Input: part model. Units: mm. Frame: model coordinates. Face numbers are marked on the shaded views. A direction names the side the tool comes from. Give positions to 0.01 mm unless a question says otherwise; leave off trailing zeros. Loops run counter-clockwise (first coordinate to the right, second up) from the corner with the lowest first, then second, coordinate; pieces in that order, holes last. Notation, with made-up numbers: (76, 9.25) - (113, 9.25) arc R26 ccw to (113, 31.25) - close; hole circle Ø5 at (40.25, 46.5). An arc over 180 degrees is marked (long way). Answer as a JSON object with one key per item and string values. Group by question number.
(1) Material intervals for L1, parallel to X at y = 26, z = 15.5; L2, parallel to X at y = 38, z = 19.5; L3, parallel to X at y = 38.2, z = 19.5, sorted ascending.
(2) Section query A-A (x = -10). Return loops of the section in (y, z), plus the area to 3 significant figures.
(3) Mould query, pull axis X, two halves, no side actions, for the marked faces 3, 4 and 5. Classes: +X half, -X half, draft (parallel to the pull), parting line (faces both ways), or undercut.
(4) Section query D-D (x = 10). Return loops of the section in (y, z).
(5) Access query for the marked faces 1 and 2. Directions: +Z, -Z, +X, -X, +Y, -Y. A direction counts if a zero-diameter tool reaches every point of the face in a straight line with its end or side. Return the directions, or none.
(6) Pin query (flat end, axial travel): P1, Ø2, axis at x = 12, z = 26.5, coming from the +Y side; P2, Ø0.8, axis at y = -4, z = 13.5, coming from the +X side; P3, Ø1.1, axis at x = 8, z = 13.5, coming from the -Y side; P4, Ø0.6, axis at x = 11.5, z = 27, coming from the -Y side. Return the tip coordinate at first contact, or that it passes through.
(7) Section query C-C (z = 19.5). Return loops of the section in (x, y), plus the area to 3 significant figures.
(8) Section query B-B (y = -18.5). Return loops of the section in (x, z), plus the area to 3 significant figures.
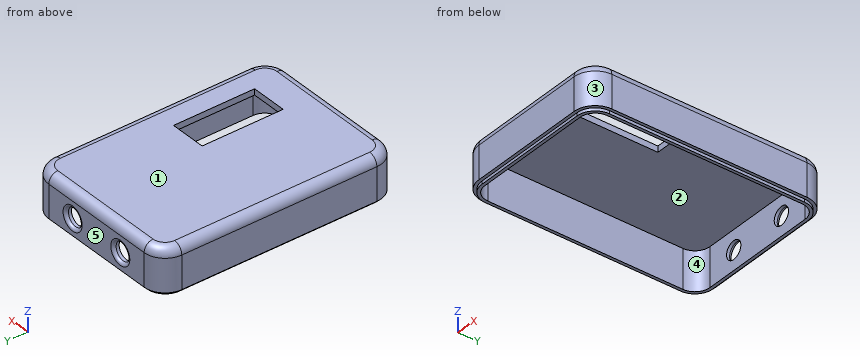
```python
from build123d import *

# Parameters (mm, degrees)
PAD002_DEPTH            = 2
PAD003_DEPTH            = 12
FILLET001_R             = 3
SKETCH006_R             = 3
POCKET002_DEPTH         = 5
PAD004_DEPTH            = 1
FILLET003_R             = 1
SKETCH018_W             = 12
SKETCH018_H             = 27
POCKET004_DEPTH         = 5
BODY001_PLACEMENT_ANGLE = 180


with BuildPart() as part:
    # Sketch003 → Pad002 (new body)
    with BuildSketch(Plane.XY):
        with BuildLine():
            Line((-27, 32.5), (-27, -32.5))
            ThreePointArc((-27, -32.5), (-24.949747, -37.449747), (-20, -39.5))
            Line((-20, -39.5), (20, -39.5))
            ThreePointArc((20, -39.5), (24.949747, -37.449747), (27, -32.5))
            Line((27, -32.5), (27, 32.5))
            ThreePointArc((27, 32.5), (24.949747, 37.449747), (20, 39.5))
            Line((20, 39.5), (-20, 39.5))
            ThreePointArc((-20, 39.5), (-24.949747, 37.449747), (-27, 32.5))
        make_face()
    extrude(amount=PAD002_DEPTH)

    # Sketch004 (on Face10 of Pad002) → Pad003 (join)
    with BuildSketch(Plane.XY.offset(2)):
        with BuildLine():
            Line((-27, 32.5), (-27, -32.5))
            ThreePointArc((-27, -32.5), (-24.949747, -37.449747), (-20, -39.5))
            Line((-20, -39.5), (20, -39.5))
            ThreePointArc((20, -39.5), (24.949747, -37.449747), (27, -32.5))
            Line((27, -32.5), (27, 32.5))
            ThreePointArc((27, 32.5), (24.949747, 37.449747), (20, 39.5))
            Line((20, 39.5), (-20, 39.5))
            ThreePointArc((-20, 39.5), (-24.949747, 37.449747), (-27, 32.5))
        make_face()
        with BuildLine():
            Line((-25, 32.5), (-25, -32.5))
            ThreePointArc((-25, -32.5), (-23.535534, -36.035534), (-20, -37.5))
            Line((-20, -37.5), (20, -37.5))
            ThreePointArc((20, -37.5), (23.535534, -36.035534), (25, -32.5))
            Line((25, -32.5), (25, 32.5))
            ThreePointArc((25, 32.5), (23.535534, 36.035534), (20, 37.5))
            Line((20, 37.5), (-20, 37.5))
            ThreePointArc((-20, 37.5), (-23.535534, 36.035534), (-25, 32.5))
        make_face(mode=Mode.SUBTRACT)
    extrude(amount=PAD003_DEPTH)

    # Fillet001
    fillet001_edges = [part.edges().sort_by_distance(p)[0] for p in [
        (0, -39.5, 0),
    ]]
    fillet(fillet001_edges, radius=FILLET001_R)

    # Sketch006 (on Face17 of Fillet001) → Pocket002 (cut)
    with BuildSketch(Plane(origin=(0, 39.5, 0), x_dir=(-1, 0, 0), z_dir=(0, 1, 0))):
        with Locations((-10, 8.5)):
            Circle(SKETCH006_R)
        with Locations((10, 8.5)):
            Circle(SKETCH006_R)
    extrude(amount=-POCKET002_DEPTH, mode=Mode.SUBTRACT)

    # Sketch008 (on Face18 of Pocket002) → Pad004 (join)
    with BuildSketch(Plane.XY.offset(14)):
        with BuildLine():
            Line((-26, 32.5), (-26, -32.5))
            ThreePointArc((-26, -32.5), (-24.242641, -36.742641), (-20, -38.5))
            Line((-20, -38.5), (20, -38.5))
            ThreePointArc((20, -38.5), (24.242641, -36.742641), (26, -32.5))
            Line((26, -32.5), (26, 32.5))
            ThreePointArc((26, 32.5), (24.242641, 36.742641), (20, 38.5))
            Line((20, 38.5), (-20, 38.5))
            ThreePointArc((-20, 38.5), (-24.242641, 36.742641), (-26, 32.5))
        make_face()
        with BuildLine():
            Line((-25, 32.5), (-25, -32.5))
            ThreePointArc((-25, -32.5), (-23.535534, -36.035534), (-20, -37.5))
            Line((-20, -37.5), (20, -37.5))
            ThreePointArc((20, -37.5), (23.535534, -36.035534), (25, -32.5))
            Line((25, -32.5), (25, 32.5))
            ThreePointArc((25, 32.5), (23.535534, 36.035534), (20, 37.5))
            Line((20, 37.5), (-20, 37.5))
            ThreePointArc((-20, 37.5), (-23.535534, 36.035534), (-25, 32.5))
        make_face(mode=Mode.SUBTRACT)
    extrude(amount=PAD004_DEPTH)

    # Fillet003
    fillet003_edges = [part.edges().sort_by_distance(p)[0] for p in [
        (-7, 39.5, 8.5),
        (13, 39.5, 8.5),
    ]]
    fillet(fillet003_edges, radius=FILLET003_R)

    # Sketch018 (on Face12 of Fillet003) → Pocket004 (cut)
    with BuildSketch(Plane(origin=(0, 0, 0), x_dir=(1, 0, 0), z_dir=(0, 0, -1))):
        with Locations((-11.4, 13.5)):
            Rectangle(SKETCH018_W, SKETCH018_H)
    extrude(amount=-POCKET004_DEPTH, mode=Mode.SUBTRACT)


with BuildPart() as part_1:
    # Body001 placement: moved
    add(part.part.moved(Location((0, 0, 28))).rotate(Axis((0, 0, 28), (0, 1, 0)), BODY001_PLACEMENT_ANGLE))


solid = part_1.part
```
Recorded:
{
 "1": {"L1": "x = -27 to -25, 25 to 27", "L2": "x = -24.33 to -13, -7 to 7, 13 to 24.33", "L3": "x = -24.06 to -13, -7 to 7, 13 to 24.06"},
 "2": {"outline": "(-39.5, 14) - (-38.5, 14) - (-38.5, 13) - (-37.5, 13) - (-37.5, 26) - (37.5, 26) - (37.5, 22.5) - (38.5, 22.5) arc R1 ccw to (39.5, 23.5) - (39.5, 25) arc R3 ccw to (36.5, 28) - (-36.5, 28) arc R3 ccw to (-39.5, 25) - close; (37.5, 13) - (38.5, 13) - (38.5, 14) - (39.5, 14) - (39.5, 15.5) arc R1 ccw to (38.5, 16.5) - (37.5, 16.5) - close", "area": "192 mm^2"},
 "3": {"face 3": "+X half", "face 4": "undercut", "face 5": "draft"},
 "4": {"outline": "(-39.5, 14) - (-38.5, 14) - (-38.5, 13) - (-37.5, 13) - (-37.5, 26) - (-27, 26) - (-27, 28) - (-36.5, 28) arc R3 ccw to (-39.5, 25) - close; (0, 26) - (37.5, 26) - (37.5, 22.5) - (38.5, 22.5) arc R1 ccw to (39.5, 23.5) - (39.5, 25) arc R3 ccw to (36.5, 28) - (0, 28) - close; (37.5, 13) - (38.5, 13) - (38.5, 14) - (39.5, 14) - (39.5, 15.5) arc R1 ccw to (38.5, 16.5) - (37.5, 16.5) - close"},
 "5": {"face 1": "+Z, +X, -X, +Y, -Y", "face 2": "-Z"},
 "6": {"P1": "stops at y = 39.46", "P2": "stops at x = 26", "P3": "stops at y = -39.5", "P4": "stops at y = -38.97"},
 "7": {"outline": "(-27, -32.5) arc R7 ccw to (-20, -39.5) - (20, -39.5) arc R7 ccw to (27, -32.5) - (27, 32.5) arc R7 ccw to (20, 39.5) - (14, 39.5) arc R1 ccw to (13, 38.5) - (13, 37.5) - (20, 37.5) arc R5 cw to (25, 32.5) - (25, -32.5) arc R5 cw to (20, -37.5) - (-20, -37.5) arc R5 cw to (-25, -32.5) - (-25, 32.5) arc R5 cw to (-20, 37.5) - (-13, 37.5) - (-13, 38.5) arc R1 ccw to (-14, 39.5) - (-20, 39.5) arc R7 ccw to (-27, 32.5) - close; (-7, 37.5) - (7, 37.5) - (7, 38.5) arc R1 ccw to (6, 39.5) - (-6, 39.5) arc R1 ccw to (-7, 38.5) - close", "area": "471 mm^2"},
 "8": {"outline": "(-27, 14) - (-26, 14) - (-26, 13) - (-25, 13) - (-25, 26) - (5.4, 26) - (5.4, 28) - (-24, 28) arc R3 ccw to (-27, 25) - close; (17.4, 26) - (25, 26) - (25, 13) - (26, 13) - (26, 14) - (27, 14) - (27, 25) arc R3 ccw to (24, 28) - (17.4, 28) - close", "area": "130 mm^2"}
}
